Verification items for this drawing (mm, ordinates from the low corner). A direction names the side the tool comes from. Coordinates: 2 decimals unless noted, no trailing zeros. Write each loop counter-clockwise with the first axis right and the second up, starting at its lowest first coordinate (ties: lowest second). Pieces come first, ordered by that corner, then holes. Notation, with made-up numbers: (-29.5, -1) -> (-8.5, -1) arc R23 cw to (-8.5, 31) -> close; hole circle Ø1 at (66, 40). An arc over 180 degrees is marked (long way). Put each result on its own line as item: value. Start each with the question number.
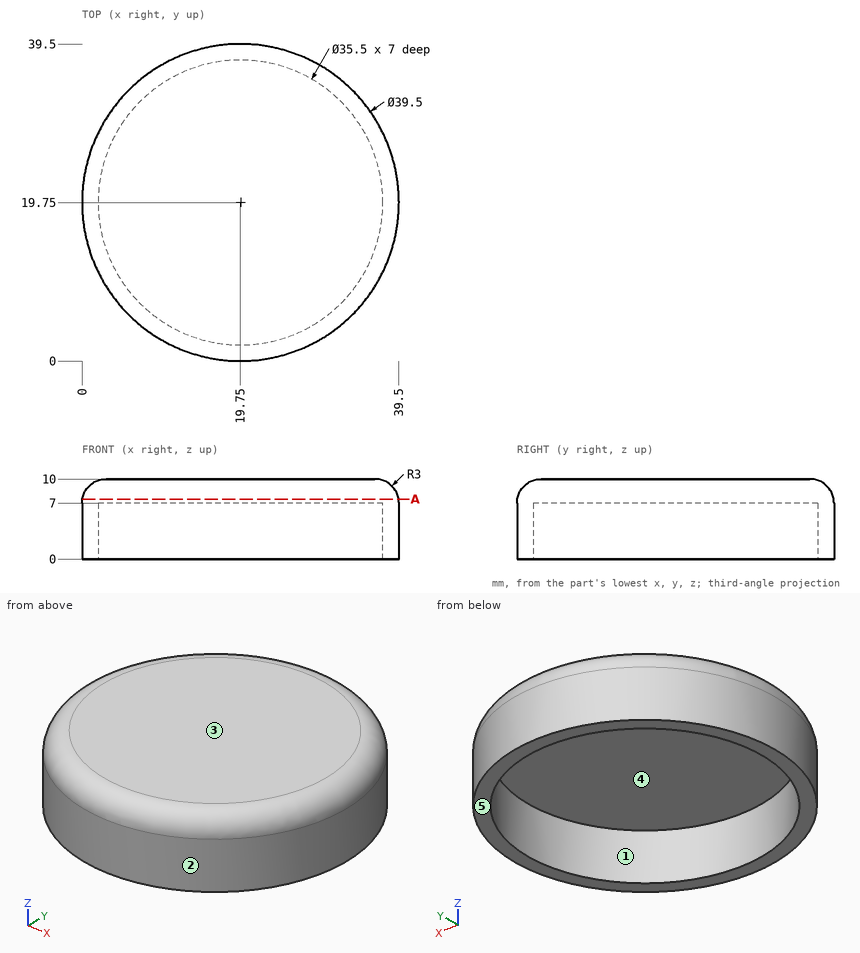
Item 1: Go/stop test with flat-tipped pins: P1, Ø1, axis at x = 12, z = 7, coming from the +Y side; P2, Ø3, axis at x = 18, y = 6.5, coming from the -Z side; P3, Ø1.5, axis at y = 13.5, z = 5.5, coming from the +X side. Record where each tip stops, or that it passes through.
Item 2: Access from +Z, -Z, +X, -X, +Y, -Y to the whole of each face (thin tool, end or side, straight path). Record for the marked faces 4 and 5.
Item 3: Mould release check, pull along X, two halves, no side actions. Record for the marked faces 1, 2 and 3: released by +X, released by -X, zero draft, split by the parting line, or undercut.
Item 4: Scan lines: line 1 along Y through (x, z) = (19.75, 2); line 2 along Z through (x, y) = (29.5, 15.5); line 3 along X through (y, z) = (17.5, 6.5). Record each from-to range of solid material in increasing order. Write a range as [from, to].
Item 5: Section check A-A, the plane z = 7.5. Enter the section's corners in (x, y).
From the geometry:
1. P1: y = 38.12
1. P2: z = 7
1. P3: x = 38.72
2. face 4: -Z
2. face 5: -Z, +X, -X, +Y, -Y
3. face 1: undercut
3. face 2: split by the parting line
3. face 3: zero draft
4. line 1: [0, 2], [37.5, 39.5]
4. line 2: [7, 10]
4. line 3: [0.13, 2.14], [37.36, 39.37]
5. outline: circle Ø39.42 at (19.75, 19.75)
